Source: three-view drawing plus pictorial views. Frame: mm from the lowest corner of the part. A direction names the side the tool comes from. Give positions to 0.01 mm unless a question says otherwise; leave off trailing zeros. Order: outer loops, then holes, each group sorted by start corner. A loop starts at its lowest first (then second) coordinate and runs counter-clockwise, first axis right, second up.
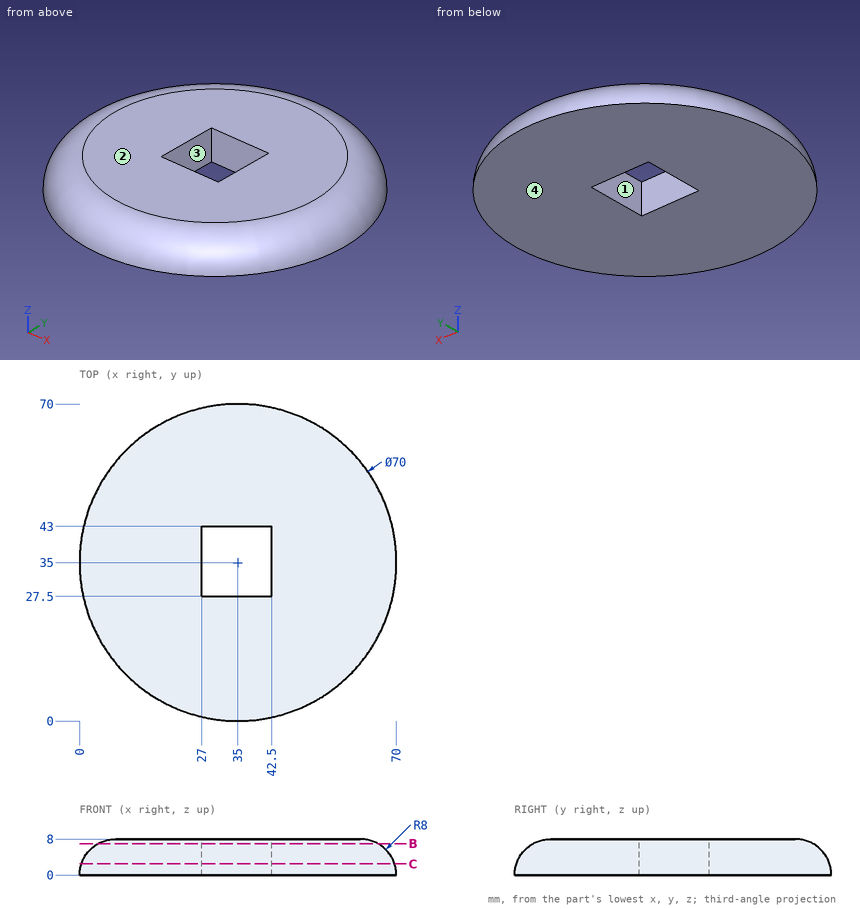
1) Ray query, L1, parallel to X at y = 33.5, z = 0.5; L2, parallel to Y at x = 41, z = 1.75; L3, parallel to Y at x = 36, z = 4.5. Return the intervals inside material, ascending.
Checks:
L1: x = 0.05 to 27, 42.5 to 69.95
L2: y = 0.71 to 27.5, 43 to 69.29
L3: y = 1.4 to 27.5, 43 to 68.6
2) First-contact query: pin 1 Ø4 at (x, z) = (34, 4) entering from -Y; pin 2 Ø2 at (y, z) = (28.5, 1.5) entering from -X; pin 3 Ø2 at (y, z) = (34.5, 4) entering from +X. Flat tips, straight axial feed; report the tip coordinate or a pass-through.
Checks:
pin 1: stops at y = 0.27
pin 2: stops at x = 0.52
pin 3: stops at x = 69.41
3) Section query C-C on z = 2.5. Output: boundary loops of the cut face in (x, y).
Checks:
outline: circle Ø69.2 at (35, 35); hole (27, 27.5) - (42.5, 27.5) - (42.5, 43) - (27, 43) - close
4) Pull-direction query (Y, two-part tool) for the marked faces 1 and 2; classes: +Y half, -Y half, draft (parallel to the pull), parting line (faces both ways), or undercut.
Checks:
face 1: undercut
face 2: draft
5) Reachability of the marked faces 3 and 4 from +Z, -Z, +X, -X, +Y, -Y: full face, straight path, thin tool, end or side. Return the list, or none.
Checks:
face 3: +Z, -Z
face 4: -Z, +X, -X, +Y, -Y
6) Section query B-B on z = 7. Output: boundary loops of the cut face in (x, y).
Checks:
outline: circle Ø61.75 at (35, 35); hole (27, 27.5) - (42.5, 27.5) - (42.5, 43) - (27, 43) - close
